Can you work these out from the model? Positions are in its coordinate system, mm. A direction names the side the tool comes from. Give positions to 0.01 mm unless a question says otherwise; leave off trailing zeros. Order: outer loops, then holes, each group sorted by start corner. A loop starts at its lowest first (then second) coordinate and runs counter-clockwise, first axis right, second up.
Item 1: I want a section at D-D, the plane x = 12.7. Write out the boundary of the cut face in (y, z) (1 decimal).
Item 2: If we mould it in two halves opening along Y, with no side actions, what happens to faces 1 (the flat face through (23.812, 13, 414)), 2 (the flat face through (13, 25.4, 411)), 3 (the cylindrical face through (12.56, 24.6, 276.23)), 4 (the flat face through (13, 0, 411))? For each: +Y half, -Y half, draft (parallel to the pull), parting line (faces both ways), or undercut.
Item 3: I want a section at C-C, the plane z = 330.2. Write out the boundary of the cut face in (x, y) (1 decimal), then the cut area to 3 significant figures.
Item 4: If I drill on line 1 along Z through (x, y) = (12.7, 24.75) (3 decimals); line 2 along Y through (x, z) = (10.75, 471), over which ranges is the centre line in solid material (lowest first)?
Item 5: I want a section at A-A, the plane y = 15.75. Write out the boundary of the cut face in (x, z).
Item 6: Which directions (+Z, -Z, +X, -X, +Y, -Y) give clear straight access to the entire face, cutting with the end or side of a thin tool? Please do faces 5 (the cylindrical face through (11.75, 24.6, 333.23)), 6 (the flat face through (1.588, 13, 414)).
Item 7: I want a section at B-B, the plane z = 285. Write out the boundary of the cut face in (x, y), then the cut area to 3 significant figures.
Item 8: I'm going to push a flat-ended pin straight in: pin 1 Ø12 at (x, y) = (12, 13) entering from -Z. Where does the tip first touch, or does it pass through?
Autodesk Inventor part; units mm, degrees
ref_plane "YZ Plane" through (0, 0, 0) normal (1, 0, 0) x (0, 1, 0)
ref_plane "XZ Plane" through (0, 0, 0) normal (0, 1, 0) x (-1, 0, 0)
ref_plane "XY Plane" through (0, 0, 0) normal (0, 0, 1) x (1, 0, 0)
sketch "Sketch1" plane through (0, 0, 0) normal (0, 0, 1) x (1, 0, 0)
  line L0 (0, 0) -> (25.4, 0)
  line L1 (25.4, 0) -> (25.4, 25.4)
  line L2 (25.4, 25.4) -> (0, 25.4)
  line L3 (0, 25.4) -> (0, 0)
  line L4 (1.5875, 1.5875) -> (23.8125, 1.5875)
  line L5 (23.8125, 1.5875) -> (23.8125, 23.8125)
  line L6 (23.8125, 23.8125) -> (1.5875, 23.8125)
  line L7 (1.5875, 23.8125) -> (1.5875, 1.5875)
  dimension "d0" = 25.4
  dimension "d1" = 25.4
  dimension "d2" = 1.5875
extrude "Extrusion1" add sketch "Sketch1" along normal blind 558.8
sketch "Sketch3" plane through (0, 25.4, 0) normal (0, 1, 0) x (1, 0, 0)
  line L0 (25.4, 0) -> (0, 0)
  line L1 (0, 0) -> (0, -558.8)
  line L2 (25.4, -558.8) -> (0, -558.8)
  line L3 (25.4, 0) -> (25.4, -558.8)
  point P0 (0, 0)
  point P1 (12.7, -279.4)
  dimension "d15" = 279.4
  dimension "d16" = 558.8
  dimension "d17" = 12.7
hole "Hole2" at (12.7, 25.4, 279.4) direction (0, -1, 0) diameter 6.35 end through all
sketch "Sketch5" plane through (0, 25.4, 0) normal (0, 1, 0) x (1, 0, 0)
  circle A0 centre (12.7, -279.4) radius 3.175
  line L0 (12.7, -279.4) -> (-12.4758, -279.4)
  point P0 (12.7, -228.6)
  point P1 (12.7, -330.2)
  dimension "d25" = 101.6
hole "Hole3" at (12.7, 25.4, 228.6) at (12.7, 25.4, 330.2) direction (0, -1, 0) diameter 6.35 end through all
sketch "Sketch7" plane through (0, 25.4, 0) normal (0, 1, 0) x (1, 0, 0)
  line L0 (0, 0) -> (0, -558.8)
  line L1 (25.4, 0) -> (25.4, -558.8)
  line L2 (25.4, 0) -> (0, 0)
  line L3 (0, 0) -> (25.4, 0)
  line L4 (0, -279.4) -> (0, 0)
  line L5 (25.4, 0) -> (25.4, -279.4)
  line L6 (0, 0) -> (25.4, 0)
  arc A0 (25.4, -279.4) -> (0, -279.4) centre (12.7, -279.4) ccw
  dimension "d41" = 279.4
extrude "Extrusion3" cut sketch "Sketch7" against normal blind 25.4
properties part number "ScissorLiftBarTop" material "Aluminum 6061"
Results list:
1. outline: (0, 266.7) - (1.6, 266.7) - (1.6, 276.2) - (0, 276.2) - close; (0, 282.6) - (1.6, 282.6) - (1.6, 327) - (0, 327) - close; (0, 333.4) - (1.6, 333.4) - (1.6, 558.8) - (0, 558.8) - close; (23.8, 266.7) - (25.4, 266.7) - (25.4, 276.2) - (23.8, 276.2) - close; (23.8, 282.6) - (25.4, 282.6) - (25.4, 327) - (23.8, 327) - close; (23.8, 333.4) - (25.4, 333.4) - (25.4, 558.8) - (23.8, 558.8) - close
2. face 1: undercut
2. face 2: +Y half
2. face 3: draft
2. face 4: -Y half
3. outline: (0, 0) - (9.5, 0) - (9.5, 1.6) - (1.6, 1.6) - (1.6, 23.8) - (9.5, 23.8) - (9.5, 25.4) - (0, 25.4) - close; (15.9, 0) - (25.4, 0) - (25.4, 25.4) - (15.9, 25.4) - (15.9, 23.8) - (23.8, 23.8) - (23.8, 1.6) - (15.9, 1.6) - close
3. area: 131 mm2
4. line 1: z = 266.7 to 276.225, 282.575 to 327.025, 333.375 to 558.8
4. line 2: y = 0 to 1.59, 23.81 to 25.4
5. outline: (0, 279.4) arc R12.7 ccw to (1.59, 273.25) - (1.59, 558.8) - (0, 558.8) - close; (23.81, 273.25) arc R12.7 ccw to (25.4, 279.4) - (25.4, 558.8) - (23.81, 558.8) - close
6. face 5: +Y, -Y
6. face 6: +Z, -Z
7. outline: (0, 0) - (25.4, 0) - (25.4, 25.4) - (0, 25.4) - close; hole (1.59, 1.59) - (23.81, 1.59) - (23.81, 23.81) - (1.59, 23.81) - close
7. area: 151 mm2
8. pin 1: passes through
